For this review, use the dimensioned drawing (mm, ordinates from the lowest corner) and the shaded views. A direction names the side the tool comes from. Give positions to 0.01 mm unless a question says otherwise; leave off trailing zeros. Write each loop counter-clockwise with the first axis right and the second up, starting at its lowest first coordinate (ties: lowest second). Pieces come first, ordered by that corner, then holes.
1) Wall thickness on line 1 along X through (y, z) = (50.5, 5.25); line 2 along X through (y, z) = (20.5, 8); line 3 along Y through (x, z) = (70.5, 10.75): over which ranges is each line inside the solid? List them lowest first.
2) We need section C-C on x = 35.5. Give the boundary of the cut face in (y, z), and give its area (3 significant figures).
3) We need section B-B on y = 43.5. Give the boundary of the cut face in (x, z), and give its area (3 significant figures).
4) We need section D-D on z = 1.75. Give the boundary of the cut face in (x, y).
5) Machinability: for the marked faces 1, 2 and 3, which of the approach directions +Z, -Z, +X, -X, +Y, -Y give a long, thin tool a straight path to every point of the face, cutting with its end or side? Answer none if there is none.
6) For P1, Ø5, axis at x = 14.5, z = 2, coming from the +Y side; P2, Ø1.5, axis at y = 12, z = 3, coming from the +X side; P3, Ø1, axis at y = 28, z = 9, coming from the -X side, all flat-tipped, find the tip position at first contact; note any pin that passes through.
7) We need section A-A on z = 9.5. Give the boundary of the cut face in (x, y), and give its area (3 significant figures).
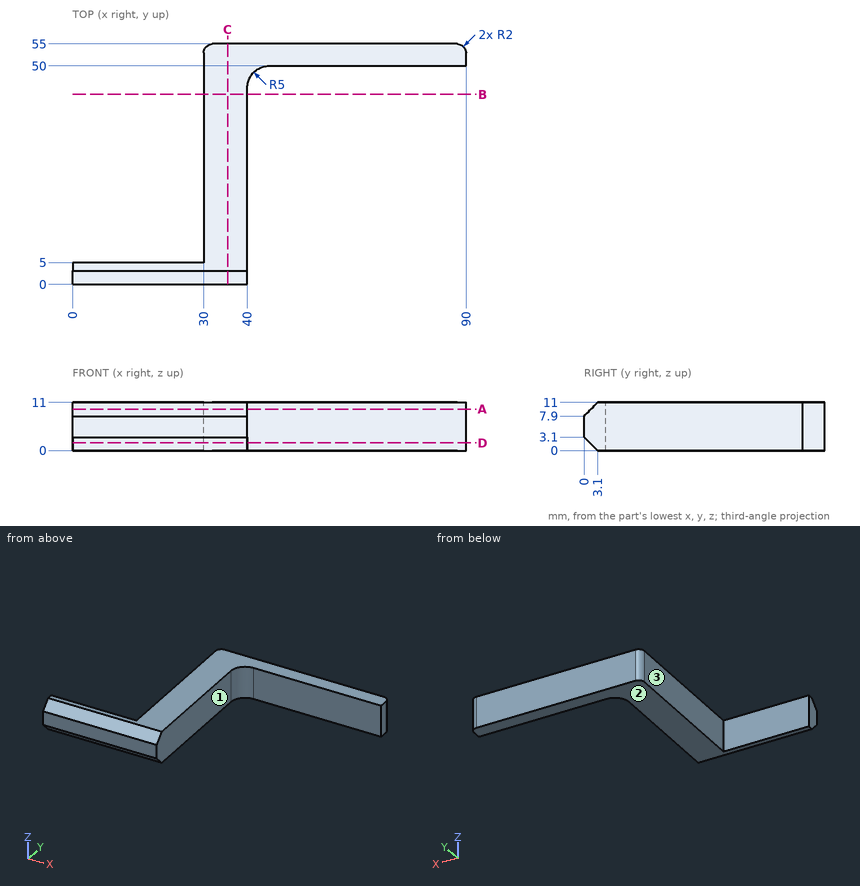
Results list:
1. line 1: x = 30 to 90
1. line 2: x = 30 to 40
1. line 3: y = 50 to 55
2. outline: (0, 3.1) - (3.1, 0) - (55, 0) - (55, 11) - (3.1, 11) - (0, 7.9) - close
2. area: 595 mm2
3. outline: (30, 0) - (40, 0) - (40, 11) - (30, 11) - close
3. area: 110 mm2
4. outline: (0, 1.35) - (40, 1.35) - (40, 45) arc R5 cw to (45, 50) - (90, 50) - (90, 53) arc R2 ccw to (88, 55) - (32, 55) arc R2 ccw to (30, 53) - (30, 5) - (0, 5) - close
5. face 1: +Z, -Z, +X, -Y
5. face 2: -Z, +X, -X, +Y, -Y
5. face 3: +Z, -Z, -X, +Y
6. P1: stops at y = 5
6. P2: stops at x = 40
6. P3: stops at x = 30
7. outline: (0, 1.6) - (40, 1.6) - (40, 45) arc R5 cw to (45, 50) - (90, 50) - (90, 53) arc R2 ccw to (88, 55) - (32, 55) arc R2 ccw to (30, 53) - (30, 5) - (0, 5) - close
7. area: 890 mm2
